```python
from build123d import *

# Parameters (mm, degrees)
SKETCH1_R           = 4.5
SKETCH1_R_2         = 2.3
BOSS_EXTRUDE1_DEPTH = 2
SKETCH2_R           = 2.5
SKETCH2_R_2         = 1.25
BOSS_EXTRUDE2_DEPTH = 10
SKETCH3_R           = 9.569639601
SKETCH3_W           = 11
SKETCH3_H           = 7.8
CUT_EXTRUDE1_DEPTH  = 10


with BuildPart() as part:
    # Sketch1 → Boss-Extrude1 (new body)
    with BuildSketch(Plane.XY):
        Circle(SKETCH1_R)
        Circle(SKETCH1_R_2, mode=Mode.SUBTRACT)
    extrude(amount=BOSS_EXTRUDE1_DEPTH)

    # Sketch2 → Boss-Extrude2 (add)
    with BuildSketch(Plane.XY.offset(2)):
        Circle(SKETCH2_R)
        Circle(SKETCH2_R_2, mode=Mode.SUBTRACT)
    extrude(amount=-BOSS_EXTRUDE2_DEPTH)

    # Sketch3 → Cut-Extrude1 (cut)
    with BuildSketch(Plane.XY.offset(2)):
        Circle(SKETCH3_R)
        Rectangle(SKETCH3_W, SKETCH3_H, mode=Mode.SUBTRACT)
    extrude(amount=-CUT_EXTRUDE1_DEPTH, mode=Mode.SUBTRACT)


solid = part.part
```
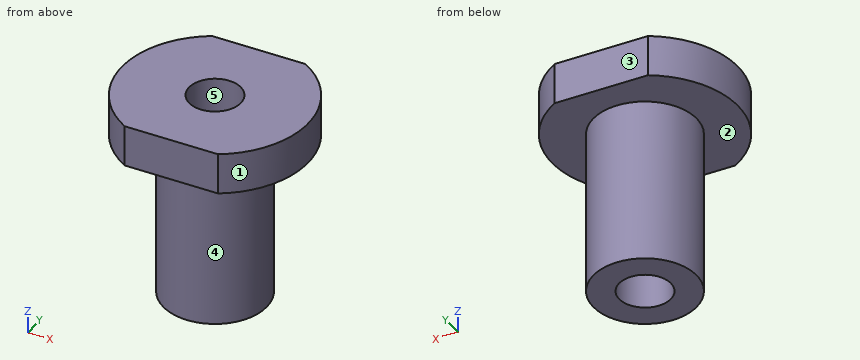
For this review, take the finished solid that the model builds, in its own axes (mm). Face numbers are marked on the shaded views. A direction names the side the tool comes from. Give positions to 0.01 mm unless a question says otherwise; leave off trailing zeros. Write each loop counter-clockwise with the first axis right and the second up, starting at its lowest first coordinate (ties: lowest second). Pieces come first, ordered by that corner, then holes.
Item 1: Take a section at B-B (x = 0). Give the boundary of the cut face in (y, z), and give its area (3 significant figures).
Item 2: Wall thickness on probe 1 along Y at (x, z) = (0, -5); probe 2 along Z at (x, y) = (-4, 1.75); probe 3 along X at (y, z) = (-2.25, 0.5): over which ranges is each line inside the solid? List them lowest first.
Item 3: Insertion check: P1, Ø4, axis at x = 0.5, z = -5.5, coming from the +Y side; P2, Ø5, axis at x = -3, z = -6, coming from the -Y side; P3, Ø1, axis at x = 0.5, y = 0.5, coming from the -Z side; P4, Ø3, axis at x = 0, y = 0, coming from the -Z side. Each pin has a flat end and moves straight along its axis. Give the tip position at first contact, or say it passes through.
Item 4: Take a section at A-A (y = 0). Give the boundary of the cut face in (x, z), and give its area (3 significant figures).
Item 5: Take a section at C-C (z = 1). Give the boundary of the cut face in (x, y) (3 decimals).
Item 6: Take a section at D-D (x = -1.5). Give the boundary of the cut face in (y, z), and give its area (3 significant figures).
Item 7: The part is to be moulded in two halves that separate along X. For the marked faces 3, 4 and 5, say which applies: +X half, -X half, draft (parallel to the pull), parting line (faces both ways), or undercut.
Item 8: Machinability: for the marked faces 1 and 2, which of the approach directions +Z, -Z, +X, -X, +Y, -Y give a long, thin tool a straight path to every point of the face, cutting with its end or side? Answer none if there is none.
Established:
1. outline: (-3.9, 0) - (-2.5, 0) - (-2.5, -8) - (-1.25, -8) - (-1.25, 2) - (-3.9, 2) - close; (1.25, -8) - (2.5, -8) - (2.5, 0) - (3.9, 0) - (3.9, 2) - (1.25, 2) - close
1. area: 30.6 mm2
2. probe 1: y = -2.5 to -1.25, 1.25 to 2.5
2. probe 2: z = 0 to 2
2. probe 3: x = -3.9 to 3.9
3. P1: stops at y = 2.5
3. P2: stops at y = -2.45
3. P3: passes through
3. P4: stops at z = -8
4. outline: (-4.5, 0) - (-2.5, 0) - (-2.5, -8) - (-1.25, -8) - (-1.25, 2) - (-4.5, 2) - close; (1.25, -8) - (2.5, -8) - (2.5, 0) - (4.5, 0) - (4.5, 2) - (1.25, 2) - close
4. area: 33.0 mm2
5. outline: (-2.245, -3.9) - (2.245, -3.9) arc R4.5 ccw to (2.245, 3.9) - (-2.245, 3.9) arc R4.5 ccw to start; hole circle Ø2.5 at (0, 0)
6. outline: (-3.9, 0) - (-2, 0) - (-2, -8) - (2, -8) - (2, 0) - (3.9, 0) - (3.9, 2) - (-3.9, 2) - close
6. area: 47.6 mm2
7. face 3: draft
7. face 4: parting line
7. face 5: undercut
8. face 1: +Z, -Z, +X
8. face 2: -Z
